Check sheet for the modelled part. Datum: model origin and axes. Units: mm. Face numbers are marked on the shaded views. Round coordinates to 2 decimals unless told otherwise and drop trailing zeros. Loops run counter-clockwise (first coordinate to the right, second up) from the corner with the lowest first, then second, coordinate; pieces in that order, holes last. Notation, with made-up numbers: (36.25, -17) -> (49.25, -17) arc R35 ccw to (49.25, 20) -> close; hole circle Ø3 at (82, 41). An arc over 180 degrees is marked (long way). One line per item, written item: value. Start each with the question number.
1. Material ranges on L1, parallel to X at y = 3, z = 0.25; L2, parallel to Y at x = -5.5, z = -6.75; L3, parallel to Z at x = -5, y = 8.25, recorded low to high.
2. Cross-section at C-C on y = 5. Record the cut outline in (x, z).
3. Release check for a two-part mould opening along Z. For the marked faces 1, 2 and 3 record: +Z half, -Z half, draft (parallel to the pull), parting line (faces both ways), or undercut.
4. Go/stop test with flat-tipped pins: pin 1 (3 mm diameter, centred on x = -2.5, y = 5.5, fed in from -Z); pin 2 (1 mm diameter, centred on x = 7.5, z = 2, fed in from +Y); pin 3 (1 mm diameter, centred on y = 6, z = 3.5, fed in from -X). Record where each tip stops, or that it passes through.
5. Cross-section at D-D on z = 10.25. Record the cut outline in (x, y).
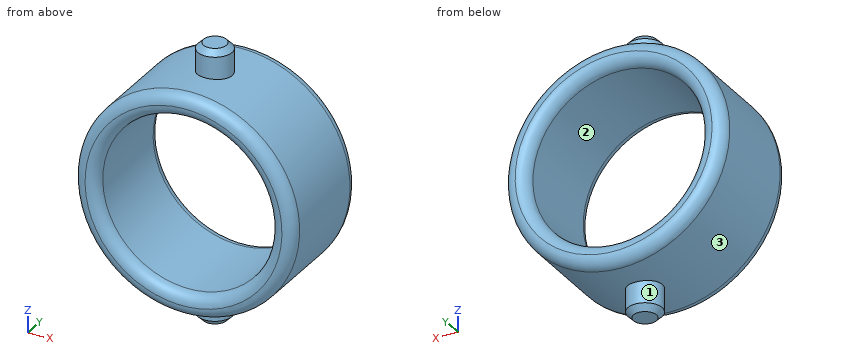
from build123d import *

# Parameters (mm, degrees)
SKETCH1_R                = 9.6
BOSS_EXTRUDE1_DEPTH      = 10
BOSS_EXTRUDE2_DEPTH      = 12
BOSS_EXTRUDE2_DEPTH_BACK = 12
SKETCH2_R                = 1.5
SKETCH3_R                = 7.6
CUT_EXTRUDE1_DEPTH       = 12
FILLET1_R                = 1
CHAMFER1_SIZE            = 0.5


with BuildPart() as part:
    # Sketch1 → Boss-Extrude1 (new body)
    with BuildSketch(Plane(origin=(0, 0, 0), x_dir=(1, 0, 0), z_dir=(0, 1, 0))):
        with Locations(Location((0, 0, 0), (0, 0, 270))):
            Circle(SKETCH1_R)
    extrude(amount=BOSS_EXTRUDE1_DEPTH)

    # Sketch2 → Boss-Extrude2 (add, two sides: drawn at the far end of the back side and taken through both)
    with BuildSketch(Plane.XY.offset(-BOSS_EXTRUDE2_DEPTH_BACK)):
        with Locations((0, 5)):
            Circle(SKETCH2_R)
    extrude(amount=BOSS_EXTRUDE2_DEPTH + BOSS_EXTRUDE2_DEPTH_BACK)

    # Sketch3 → Cut-Extrude1 (cut)
    with BuildSketch(Plane(origin=(0, 10, 0), x_dir=(1, 0, 0), z_dir=(0, 1, 0))):
        with Locations(Location((0, 0, 0), (0, 0, 270))):
            Circle(SKETCH3_R)
    extrude(amount=-CUT_EXTRUDE1_DEPTH, mode=Mode.SUBTRACT)

    # Fillet1
    fillet1_edges = [part.edges().sort_by_distance(p)[0] for p in [
        (0, 0, -7.6),
        (0, 10, -7.6),
        (0, 0, -9.6),
        (0, 10, -9.6),
    ]]
    fillet(fillet1_edges, radius=FILLET1_R - 0.0001)  # a hair under: the kernel refuses the full size

    # Chamfer1
    chamfer1_edges = [part.edges().sort_by_distance(p)[0] for p in [
        (-1.5, 5, -12),
        (-1.5, 5, 12),
    ]]
    chamfer(chamfer1_edges, length=CHAMFER1_SIZE)


solid = part.part
Taken from the geometry:
1. L1: x = -9.6 to -7.6, 7.6 to 9.6
1. L2: y = 0.01 to 9.99
1. L3: z = -8.2 to -5.72, 5.72 to 8.2
2. outline: (-1.5, -11.5) -> (-1, -12) -> (1, -12) -> (1.5, -11.5) -> (1.5, -9.48) arc R9.6 ccw to (1.5, 9.48) -> (1.5, 11.5) -> (1, 12) -> (-1, 12) -> (-1.5, 11.5) -> (-1.5, 9.48) arc R9.6 ccw to (-1.5, -9.48) -> close; hole circle Ø15.2 at (0, 0)
3. face 1: draft
3. face 2: undercut
3. face 3: parting line
4. pin 1: stops at z = -11.95
4. pin 2: stops at y = 9.94
4. pin 3: stops at x = -9.12
5. outline: circle Ø3 at (0, 5)
